Can you work these out from the model? Positions are in its coordinate system, mm. A direction names the side the tool comes from. Coordinates: 2 decimals unless noted, no trailing zeros. Order: outer loops, then holes, each group sorted by start corner. A loop starts at its lowest first (then second) coordinate and runs counter-clockwise, first axis right, second up. Notation, with made-up numbers: (11, 22.25) -> (43, 22.25) arc R32 ccw to (43, 55.25) -> close; hole circle Ø9 at (10, -17). An arc over 180 degrees is marked (long way). Answer as CSV lines item,"result".
from build123d import *

# Parameters (mm, degrees)
BOSS_EXTRUDE1_DEPTH = 7
SKETCH4_W           = 8
SKETCH4_H           = 7
CUT_EXTRUDE5_DEPTH  = 5.473756706
CUT_EXTRUDE6_REACH  = 28.532
SKETCH7_R           = 1.75
FILLET3_R           = 1


with BuildPart() as part:
    # Sketch1 → Boss-Extrude1 (new body)
    with BuildSketch(Plane(origin=(0, 0, 0), x_dir=(1, 0, 0), z_dir=(0, 1, 0))):
        with BuildLine():
            Line((0, 0), (-8, 0))
            Line((-8, 0), (-8, 3.5))
            Line((-8, 3.5), (-2.480268528, 3.5))
            ThreePointArc((-2.480268528, 3.5), (8.5, 8.973756706), (19.480268528, 3.5))
            Line((19.480268528, 3.5), (25, 3.5))
            Line((25, 3.5), (25, 0))
            Line((25, 0), (17, 0))
            ThreePointArc((17, 0), (8.5, 4.973756706), (0, 0))
        make_face()
    extrude(amount=BOSS_EXTRUDE1_DEPTH)

    # Sketch4 → Cut-Extrude5 (cut)
    with BuildSketch(Plane(origin=(0, 0, -8.973756706), x_dir=(-1, 0, 0), z_dir=(0, 0, -1))):
        with Locations((-21, 3.5)):
            Rectangle(SKETCH4_W, SKETCH4_H)
        with Locations((4, 3.5)):
            Rectangle(SKETCH4_W, SKETCH4_H)
    extrude(amount=-CUT_EXTRUDE5_DEPTH, mode=Mode.SUBTRACT)

    # Sketch7 → Cut-Extrude6 (cut, up to next)
    with BuildSketch(Plane(origin=(0, 0, -3.5), x_dir=(-1, 0, 0), z_dir=(0, 0, -1)), mode=Mode.PRIVATE) as cut_extrude6_sk1:
        with Locations((-20.999991214, 3.5)):
            Circle(SKETCH7_R)
    cut_extrude6_tool1 = extrude(cut_extrude6_sk1.sketch, amount=-CUT_EXTRUDE6_REACH, mode=Mode.PRIVATE) & part.part
    # Sketch7 → Cut-Extrude6 (cut, up to next)
    with BuildSketch(Plane(origin=(0, 0, -3.5), x_dir=(-1, 0, 0), z_dir=(0, 0, -1)), mode=Mode.PRIVATE) as cut_extrude6_sk2:
        with Locations((4.000006362, 3.511008166)):
            Circle(SKETCH7_R)
    cut_extrude6_tool2 = extrude(cut_extrude6_sk2.sketch, amount=-CUT_EXTRUDE6_REACH, mode=Mode.PRIVATE) & part.part
    add(cut_extrude6_tool1.solids().sort_by_distance((20.999991, 3.5, -3.5))[0], mode=Mode.SUBTRACT)
    add(cut_extrude6_tool2.solids().sort_by_distance((-4.000006, 3.511008, -3.5))[0], mode=Mode.SUBTRACT)

    # Fillet3
    fillet3_edges = [part.edges().sort_by_distance(p)[0] for p in [
        (-8, 3.5, -3.5),
        (25, 3.5, -3.5),
        (17, 3.5, -6.031739867),
        (17, 3.5, -3.5),
        (0, 3.5, -6.031739867),
        (0, 3.5, -3.5),
    ]]
    fillet(fillet3_edges, radius=FILLET3_R)


solid = part.part
Q1. Imagine slicing it at A-A (x = -4). List the corners of the cut face in (y, z) for me.
Solution:
outline,"(0, -3.5) -> (1.76, -3.5) -> (1.76, 0) -> (0, 0) -> close; (5.26, -3.5) -> (7, -3.5) -> (7, 0) -> (5.26, 0) -> close"
Q2. Which directions (+Z, -Z, +X, -X, +Y, -Y) give clear straight access to the entire face, cutting with the end or side of a thin tool? Please do faces 5 (the flat face through (-6, 3, -3.5)), 6 (the flat face through (17, 3, -5)), 7 (the flat face through (9, 0, -6)).
Solution:
face 5,"-Z, -X, +Y, -Y"
face 6,"-Z, +X, +Y, -Y"
face 7,"+Z, -Z, +X, -X, -Y"
Q3. For P1, Ø1.1, axis at y = 4.5, z = -5, coming from the -X side, with a flat end and sliding along its axis, tell me the tip position at first contact or that it passes through.
Solution:
P1,"x = 0"
Q4. Imagine slicing it at D-D (x = 8.5). List the corners of the cut face in (y, z) for me, and give its area (3 significant figures).
Solution:
outline,"(0, -8.97) -> (7, -8.97) -> (7, -4.97) -> (0, -4.97) -> close"
area,"28.0 mm2"
Q5. Imagine slicing it at B-B (y = 3). List the corners of the cut face in (x, z) for me, and give its area (3 significant figures).
Solution:
outline,"(-8, -2.5) arc R1 ccw to (-7, -3.5) -> (-5.67, -3.5) -> (-5.67, 0) -> (-8, 0) -> close; (-2.33, -3.5) -> (-1, -3.5) arc R1 cw to (0, -4.5) -> (0, -5.53) arc R1 ccw to (0.41, -6.34) arc R13.75 ccw to (16.59, -6.34) arc R1 ccw to (17, -5.53) -> (17, -4.5) arc R1 cw to (18, -3.5) -> (19.32, -3.5) -> (19.32, 0) -> (17, 0) arc R9.75 cw to (0, 0) -> (-2.33, 0) -> close; (22.68, -3.5) -> (24, -3.5) arc R1 ccw to (25, -2.5) -> (25, 0) -> (22.68, 0) -> close"
area,"109 mm2"
Q6. We'd pull the mould along X, two halves only. Please class faces 1 (the flat face through (-8, 3, -1)), 2 (the cylindrical face through (8.645, 3.451, -4.973)), 3 (the cylindrical face through (-5.6, 2.8, -1.8)), 4 (the cylindrical face through (16.89, 3.45, -5.99)): pulls with the +X half, pulls with the -X half, needs draft (parallel to the pull), parting line crosses it, or undercut.
Solution:
face 1,"pulls with the -X half"
face 2,"undercut"
face 3,"undercut"
face 4,"pulls with the +X half"
Q7. If I drill on line 1 (Z direction, x = 18, y = 6); line 2 (X direction, y = 2.75, z = -1); line 3 (X direction, y = 5, z = -1.5), over which ranges is the centre line in solid material (lowest first)?
Solution:
line 1,"-3.5 to 0"
line 2,"-8 to -5.58, -2.42 to 0.65, 16.35 to 19.42, 22.58 to 25"
line 3,"-8 to -4.92, -3.08 to 1.04, 15.96 to 20.1, 21.9 to 25"
Q8. Imagine slicing it at C-C (z = -1). List the corners of the cut face in (x, y) for me, and give its area (3 significant figures).
Solution:
outline,"(-8, 0) -> (0.65, 0) -> (0.65, 7) -> (-8, 7) -> close; (16.35, 0) -> (25, 0) -> (25, 7) -> (16.35, 7) -> close; hole circle Ø3.5 at (-4, 3.51); hole circle Ø3.5 at (21, 3.5)"
area,"102 mm2"
